```python
from build123d import *

# Parameters (mm, degrees)
RESSALTO_EXTRUS_O1_DEPTH = 40
FILETE1_R                = 10
ESBO_O3_R                = 2.5
CORTE_EXTRUS_O1_DEPTH    = 60


with BuildPart() as part:
    # Esboço1 → Ressalto-extrusão1 (new body)
    with BuildSketch(Plane.XY):
        Polygon((0, 0), (0, 50), (10, 50), (10, 10), (40, 10), (40, 50), (50, 50), (50, 0), align=None)
    extrude(amount=RESSALTO_EXTRUS_O1_DEPTH)

    # Filete1
    filete1_edges = [part.edges().sort_by_distance(p)[0] for p in [
        (0, 0, 20),
        (50, 0, 20),
    ]]
    fillet(filete1_edges, radius=FILETE1_R)

    # Esboço3 → Corte-extrusão1 (cut)
    with BuildSketch(Plane.ZY):
        with Locations((-0.627602125, 39.325673362)):
            Circle(ESBO_O3_R)
        with Locations((9.138766469, 37.17670978)):
            Circle(ESBO_O3_R)
        with Locations((6.989802887, 27.410341185)):
            Circle(ESBO_O3_R)
        with Locations((-2.776565708, 29.559304768)):
            Circle(ESBO_O3_R)
    extrude(amount=-CORTE_EXTRUS_O1_DEPTH, mode=Mode.SUBTRACT)


solid = part.part
```
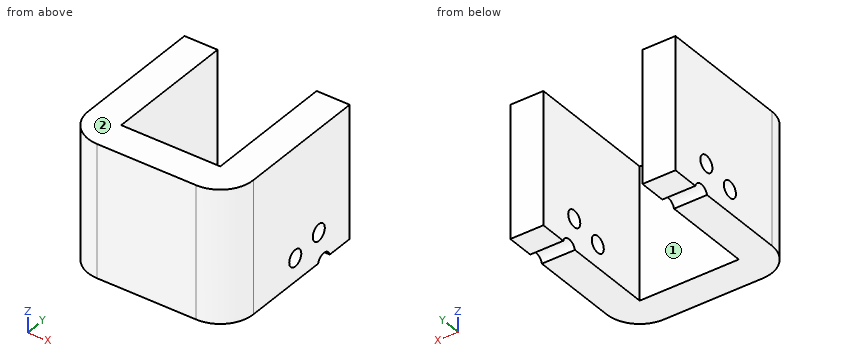
Can you work these out from the model? Positions are in its coordinate system, mm. Face numbers are marked on the shaded views. A direction names the side the tool comes from. Round coordinates to 2 decimals unless told otherwise and drop trailing zeros. Loops run counter-clockwise (first coordinate to the right, second up) from the corner with the lowest first, then second, coordinate; pieces in that order, holes last. Notation, with made-up numbers: M -20.5,69 L 36.5,69 A18 ccw 36.5,94 Z; hole C 11,61 d8. An arc over 180 degrees is marked long. Write item = value, one per line. Start each with the question number.
(1) Which directions (+Z, -Z, +X, -X, +Y, -Y) give clear straight access to the entire face, cutting with the end or side of a thin tool? Please do the marked faces 1 and 2.
(2) Suppose I cut it at B-B on z = 25. Write out the boundary of the cut face in (x, y), plus the area to 3 significant figures.
(3) I need wall thicknesses on line 1 along X through (y, z) = (40, 16.5); line 2 along Y through (x, z) = (13.5, 30); line 3 along Z through (x, y) = (3, 29). Which ranges of each line are inside material? Lowest first, please.
(4) I'm going to push flat-ended pins straight in: P1, Ø15, axis at x = 23.5, z = 10.5, coming from the +Y side; P2, Ø1.5, axis at x = 42, z = 8, coming from the -Y side. Where does each tip first touch, or does it pass through?
(5) Suppose I cut it at D-D on z = 7.5. Write out the boundary of the cut face in (x, y).
(6) Suppose I cut it at A-A on y = 12.5. Write out the boundary of the cut face in (x, z), plus the area to 3 significant figures.
(7) Suppose I cut it at C-C on x = 5. Write out the boundary of the cut face in (y, z).
Answer block:
q1.face_1 = +Z, -Z, +Y
q1.face_2 = +Z, +X, -X, +Y, -Y
q2.outline = M 0,10 A10 ccw 10,0 L 40,0 A10 ccw 50,10 L 50,50 L 40,50 L 40,10 L 10,10 L 10,50 L 0,50 Z
q2.area = 1,260 mm²
q3.line_1 = 0 to 10, 40 to 50
q3.line_2 = 0 to 10
q3.line_3 = 0 to 5.06, 8.92 to 40
q4.P1 = 10
q4.P2 = 0.08
q5.outline = M 0,10 A10 ccw 10,0 L 40,0 A10 ccw 50,10 L 50,24.96 L 40,24.96 L 40,10 L 10,10 L 10,24.96 L 0,24.96 Z; M 0,29.86 L 10,29.86 L 10,35.29 L 0,35.29 Z; M 0,39.06 L 10,39.06 L 10,50 L 0,50 Z; M 40,29.86 L 50,29.86 L 50,35.29 L 40,35.29 Z; M 40,39.06 L 50,39.06 L 50,50 L 40,50 Z
q6.outline = M 0,0 L 10,0 L 10,40 L 0,40 Z; M 40,0 L 50,0 L 50,40 L 40,40 Z
q6.area = 800 mm²
q7.outline = M 1.34,0 L 36.91,0 A2.5 cw 41.75,0 L 50,0 L 50,40 L 1.34,40 Z; hole C 27.41,6.99 d5; hole C 37.18,9.14 d5
